Autodesk Inventor part; units mm, degrees
ref_plane "YZ Plane" through (0, 0, 0) normal (1, 0, 0) x (0, 1, 0)
ref_plane "XZ Plane" through (0, 0, 0) normal (0, 1, 0) x (-1, 0, 0)
ref_plane "XY Plane" through (0, 0, 0) normal (0, 0, 1) x (1, 0, 0)
sketch "Sketch1" plane through (0, 0, 0) normal (0, 0, 1) x (1, 0, 0)
  line L0 (0, 0) -> (186, 0)
  line L1 (186, 0) -> (186, 40)
  line L2 (186, 40) -> (0, 40)
  line L3 (0, 40) -> (0, 0)
  dimension "d0" = 186
  dimension "d1" = 40
extrude "Extrusion1" add sketch "Sketch1" along normal blind 5
sketch "Sketch2" plane through (0, 0, 5) normal (0, 0, 1) x (1, 0, 0)
  line L0 (186, 40) -> (0, 40)
  line L1 (0, 0) -> (186, 0)
  line L2 (0, 40) -> (0, 0)
  point P0 (43, 30)
  point P1 (43, 10)
  dimension "d4" = 10
  dimension "d6" = 43
  dimension "d40" = 20
  dimension "d41" = 10
hole "Hole1" at (43, 30, 5) at (43, 10, 5) direction (0, 0, -1) diameter 4.5 end through all
pattern_linear "Rectangular Pattern1" count 3 spacing 50 along (1, 0, 0) of "Hole1"
sketch "Sketch3" plane through (0, 0, 5) normal (0, 0, 1) x (1, 0, 0)
  line L0 (186, 40) -> (0, 40)
  line L1 (0, 40) -> (0, 0)
  line L2 (186, 0) -> (186, 40)
  point P0 (58.4348, 20)
  point P1 (127.5652, 9)
  dimension "d17" = 70
  dimension "d18" = 20
  dimension "d19" = 11
  dimension "d20" = 58.4348
  dimension "d21" = 58.4348
hole "Hole2" at (58.4348, 20, 5) at (127.5652, 9, 5) direction (0, 0, -1) diameter 4.5 end through all
sketch "Sketch4" plane through (0, 0, 5) normal (0, 0, 1) x (1, 0, 0)
  line L0 (186, 40) -> (0, 40)
  line L1 (0, 0) -> (186, 0)
  line L2 (0, 40) -> (0, 0)
  line L3 (186, 0) -> (186, 40)
  point P0 (12.5, 32.5)
  point P1 (12.5, 7.5)
  point P2 (173.5, 32.5)
  point P3 (173.5, 7.5)
  dimension "d29" = 7.5
  dimension "d30" = 7.5
  dimension "d31" = 12.5
  dimension "d32" = 12.5
hole "Hole3" at (12.5, 32.5, 5) at (12.5, 7.5, 5) at (173.5, 32.5, 5) at (173.5, 7.5, 5) direction (0, 0, -1) diameter 4.5 end through all
sketch "Sketch5" plane through (0, 0, 5) normal (0, 0, 1) x (1, 0, 0)
  line L0 (186, 40) -> (0, 40)
  line L1 (186, 0) -> (186, 40)
  line L2 (0, 40) -> (0, 0)
  point P0 (25, 35)
  point P1 (161, 35)
  dimension "d42" = 5
  dimension "d43" = 25
  dimension "d44" = 25
hole "Hole4" at (25, 35, 5) at (161, 35, 5) direction (0, 0, -1) diameter 3 end through all
properties part number "Top_Slider Piece 1_3 Lanes" material "Wood (Oak)"
The model under review builds one solid part; all positions refer to its coordinate system, in mm. Round coordinates to 2 decimals unless told otherwise and drop trailing zeros. Order: outer loops, then holes, each group sorted by start corner. A loop starts at its lowest first (then second) coordinate and runs counter-clockwise, first axis right, second up. Notation, with made-up numbers: (21.25, 67) - (50.25, 67) arc R26 cw to (50.25, 81) - close; hole circle Ø9 at (45, 19.5). An arc over 180 degrees is marked (long way). Use one line per item in the form item = value.
Q1. Mouldability with a two-part tool opening along X and no side actions: class faces 1 (the flat face through (0, 20, 2)), 2 (the cylindrical face through (95.196, 30.488, 2.465)), 3 (the flat face through (92, 20, 5)) as pulls with the +X half, pulls with the -X half, needs draft (parallel to the pull), parting line crosses it, or undercut.
Response values:
face_1 = pulls with the -X half
face_2 = undercut
face_3 = needs draft
Q2. Add section A-A on x = 93. Give the boundary of the cut face in (y, z).
Response values:
outline = (0, 0) - (7.75, 0) - (7.75, 5) - (0, 5) - close; (12.25, 0) - (27.75, 0) - (27.75, 5) - (12.25, 5) - close; (32.25, 0) - (40, 0) - (40, 5) - (32.25, 5) - close
Q3. To check wall thickness, follow line 1 (Y direction, x = 12.5, z = 2.25); line 2 (X direction, y = 35, z = 3.7); line 3 (X direction, y = 30, z = 3.6). State the ranges of each line that lie inside material, in increasing order.
Response values:
line_1 = 0 to 5.25, 9.75 to 30.25, 34.75 to 40
line_2 = 0 to 23.5, 26.5 to 159.5, 162.5 to 186
line_3 = 0 to 40.75, 45.25 to 90.75, 95.25 to 140.75, 145.25 to 186
Q4. Clearance check with a flat-ended pin moving along its axis: P1, Ø2.5, axis at x = 143, y = 10, coming from the +Z side. State where the tip first meets the part, or that it passes through.
Response values:
P1 = through
Q5. Add section B-B on z = 3.9. Give the number of separate pieces and of enclosed holes in the cut face, then the cut area to 4 significant figures.
Response values:
separate_pieces = 1
enclosed_holes = 14
area = 7,235 mm^2
